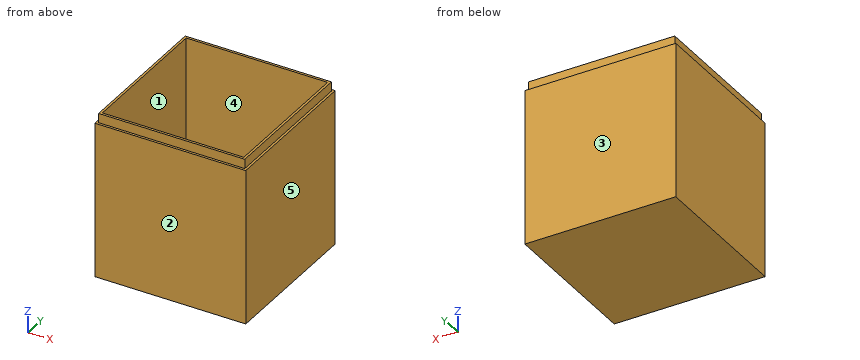
```python
from build123d import *

# Parameters (mm, degrees)
SKETCH1_W           = 81.28
SKETCH1_H           = 81.28
BOSS_EXTRUDE1_DEPTH = 88.9
SHELL1_T            = -2.54
SKETCH2_W           = 91.781641856
SKETCH2_H           = 86.951733082
SKETCH2_W_2         = 78.74
SKETCH2_H_2         = 78.74
CUT_EXTRUDE1_DEPTH  = 5.08


with BuildPart() as part:
    # Sketch1 → Boss-Extrude1 (new body)
    with BuildSketch(Plane.XY):
        Rectangle(SKETCH1_W, SKETCH1_H)
    extrude(amount=BOSS_EXTRUDE1_DEPTH)

    # Shell1
    shell1_openings = [part.faces().sort_by_distance(p)[0] for p in [
        (0, 0, 88.9),
    ]]
    offset(amount=SHELL1_T, openings=shell1_openings, kind=Kind.INTERSECTION)

    # Sketch2 → Cut-Extrude1 (cut)
    with BuildSketch(Plane.XY.offset(88.9)):
        Rectangle(SKETCH2_W, SKETCH2_H)
        Rectangle(SKETCH2_W_2, SKETCH2_H_2, mode=Mode.SUBTRACT)
    extrude(amount=-CUT_EXTRUDE1_DEPTH, mode=Mode.SUBTRACT)


solid = part.part
```
Input: part model. Units: mm. Frame: model coordinates. Face numbers are marked on the shaded views. A direction names the side the tool comes from. Round coordinates to 2 decimals unless told otherwise and drop trailing zeros. Loops run counter-clockwise (first coordinate to the right, second up) from the corner with the lowest first, then second, coordinate; pieces in that order, holes last. Notation, with made-up numbers: M -25.75,-21.75 L -16.75,-21.75 A20 ccw -16.75,-5.75 Z; hole C -24.5,35.5 d9. An arc over 180 degrees is marked long. Answer in a Markdown table with one row per item. Add a question column.
1. Set-up query: the marked faces 1 and 2. Return all of +Z, -Z, +X, -X, +Y, -Y with unobstructed straight access to the full face (end or side cutting, diameter ignored); none if empty.
2. Contact query for flat-ended pins moving along their axis: pin 1 (4 mm diameter, centred on x = 8, z = 85.5, fed in from +Y); pin 2 (2.5 mm diameter, centred on x = 3, z = 86.5, fed in from -Y); pin 3 (5 mm diameter, centred on x = 6, y = -20, fed in from +Z). Output: stop coordinate, or through.
3. Ray query, probe 1 along Y at (x, z) = (10, 47.5); probe 2 along Z at (x, y) = (-3.5, 11). Return the intervals inside material, ascending.
4. Section A-A (z = 41.5). Output: boundary loops of the cut face in (x, y), and give its area (3 significant figures).
5. Section B-B (y = 16.5). Output: boundary loops of the cut face in (x, z), and give its area (3 significant figures).
6. Mould query, pull axis Y, two halves, no side actions, for the marked faces 3, 4 and 5. Classes: released by +Y, released by -Y, zero draft, split by the parting line, or undercut.
Values follow:
| question | item | result |
|---|---|---|
| 1 | face 1 | +Z |
| 1 | face 2 | +Z, -Z, +X, -X, -Y |
| 2 | pin 1 | y = 40.64 |
| 2 | pin 2 | y = -39.37 |
| 2 | pin 3 | z = 2.54 |
| 3 | probe 1 | -40.64 to -38.1, 38.1 to 40.64 |
| 3 | probe 2 | 0 to 2.54 |
| 4 | outline | M -40.64,-40.64 L 40.64,-40.64 L 40.64,40.64 L -40.64,40.64 Z; hole M -38.1,-38.1 L 38.1,-38.1 L 38.1,38.1 L -38.1,38.1 Z |
| 4 | area | 800 mm^2 |
| 5 | outline | M -40.64,0 L 40.64,0 L 40.64,83.82 L 39.37,83.82 L 39.37,88.9 L 38.1,88.9 L 38.1,2.54 L -38.1,2.54 L -38.1,88.9 L -39.37,88.9 L -39.37,83.82 L -40.64,83.82 Z |
| 5 | area | 632 mm^2 |
| 6 | face 3 | released by +Y |
| 6 | face 4 | undercut |
| 6 | face 5 | zero draft |
